Geometry check sheet. Reference: the model listing, model coordinates, mm. Coordinates: 2 decimals unless noted, no trailing zeros. Order: outer loops, then holes, each group sorted by start corner. A loop starts at its lowest first (then second) coordinate and runs counter-clockwise, first axis right, second up. Notation, with made-up numbers: M 16.5,-35 L 60.5,-35 A9 ccw 60.5,-31 Z; hole C -16,77 d8. An arc over 180 degrees is marked long. Use CSV: the item, a comma, the result in double quotes. Start each with the question number.
Autodesk Inventor part; units mm, degrees
ref_plane "YZ Plane" through (0, 0, 0) normal (1, 0, 0) x (0, 1, 0)
ref_plane "XZ Plane" through (0, 0, 0) normal (0, 1, 0) x (-1, 0, 0)
ref_plane "XY Plane" through (0, 0, 0) normal (0, 0, 1) x (1, 0, 0)
sketch "Sketch1" plane through (0, 0, 0) normal (0, 0, 1) x (1, 0, 0)
  line L0 (0, 0) -> (25.4, 0)
  line L1 (25.4, 0) -> (25.4, 25.4)
  line L2 (25.4, 25.4) -> (0, 25.4)
  line L3 (0, 25.4) -> (0, 0)
  line L4 (1.5875, 23.8125) -> (23.8125, 23.8125)
  line L5 (23.8125, 23.8125) -> (23.8125, 1.5875)
  line L6 (23.8125, 1.5875) -> (1.5875, 1.5875)
  line L7 (1.5875, 1.5875) -> (1.5875, 23.8125)
  dimension "d0" = 25.4
  dimension "d2" = 25.4
  dimension "d3" = 1.5875
extrude "Extrusion1" add sketch "Sketch1" along normal blind 495.3
sketch "Sketch2" plane through (0, 25.4, 0) normal (0, 1, 0) x (1, 0, 0)
  line L0 (25.4, 0) -> (0, 0)
  line L1 (0, 0) -> (0, -495.3)
  line L2 (25.4, -495.3) -> (0, -495.3)
  line L3 (25.4, 0) -> (25.4, -495.3)
  line L4 (25.4, -495.3) -> (0, -469.9)
  line L5 (25.4, 0) -> (0, -25.4)
  dimension "d6" = 135
  dimension "d7" = 45
extrude "Extrusion2" cut sketch "Sketch2" against normal blind 495.3 contours L5 L1 L0 | L2 L1 L4
sketch "Sketch3" plane through (25.4, 0, 0) normal (0, -1, 0) x (1, 0, 0)
  circle A0 centre (-12.7, 69.85) radius 3.3782
  circle A1 centre (-12.7, 47.625) radius 3.3782
  circle A2 centre (-12.7, 425.45) radius 3.3782
  circle A3 centre (-12.7, 447.675) radius 3.3782
  point P0 (-25.4, 0)
extrude "Extrusion3" cut sketch "Sketch3" against normal blind 25.4
sketch "Sketch4" plane through (0, 0, 25.4) normal (-1, 0, 0) x (0, 0, 1)
  circle A0 centre (431.8, 12.7) radius 3.3782
  circle A1 centre (381, 12.7) radius 3.3782
  circle A2 centre (12.7, 12.7) radius 3.3782
  circle A3 centre (63.5, 12.7) radius 3.3782
  point P0 (-25.4, 0)
extrude "Extrusion4" cut sketch "Sketch4" against normal blind 25.4
properties part number "Square Tube 2" material "Aluminum 6061"
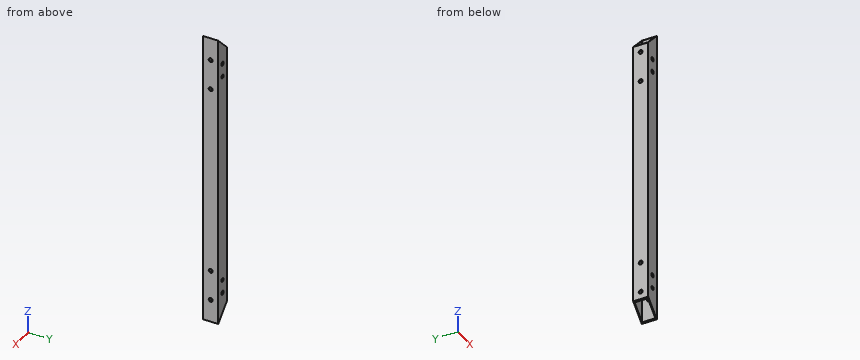
1) Gauge pin test, flat ends, axial feed: P1, Ø8, axis at y = 12.7, z = 406.4, coming from the +X side; P2, Ø12, axis at x = 3.5, y = 9.5, coming from the +Z side. Record the tip position at first contact, or that the pin passes through.
2) Section check A-A on z = 232.5. Record the boundary of the cut face in (x, y).
3) Material ranges on line 1 along Y through (x, z) = (4.5, 315); line 2 along Y through (x, z) = (1, 88.9), recorded low to high.
Results are:
1,P1,"stops at x = 25.4"
1,P2,"stops at z = 471.49"
2,outline,"M 0,0 L 25.4,0 L 25.4,25.4 L 0,25.4 Z; hole M 1.59,1.59 L 23.81,1.59 L 23.81,23.81 L 1.59,23.81 Z"
3,line 1,"y = 0 to 1.59, 23.81 to 25.4"
3,line 2,"y = 0 to 9.32, 16.08 to 25.4"
